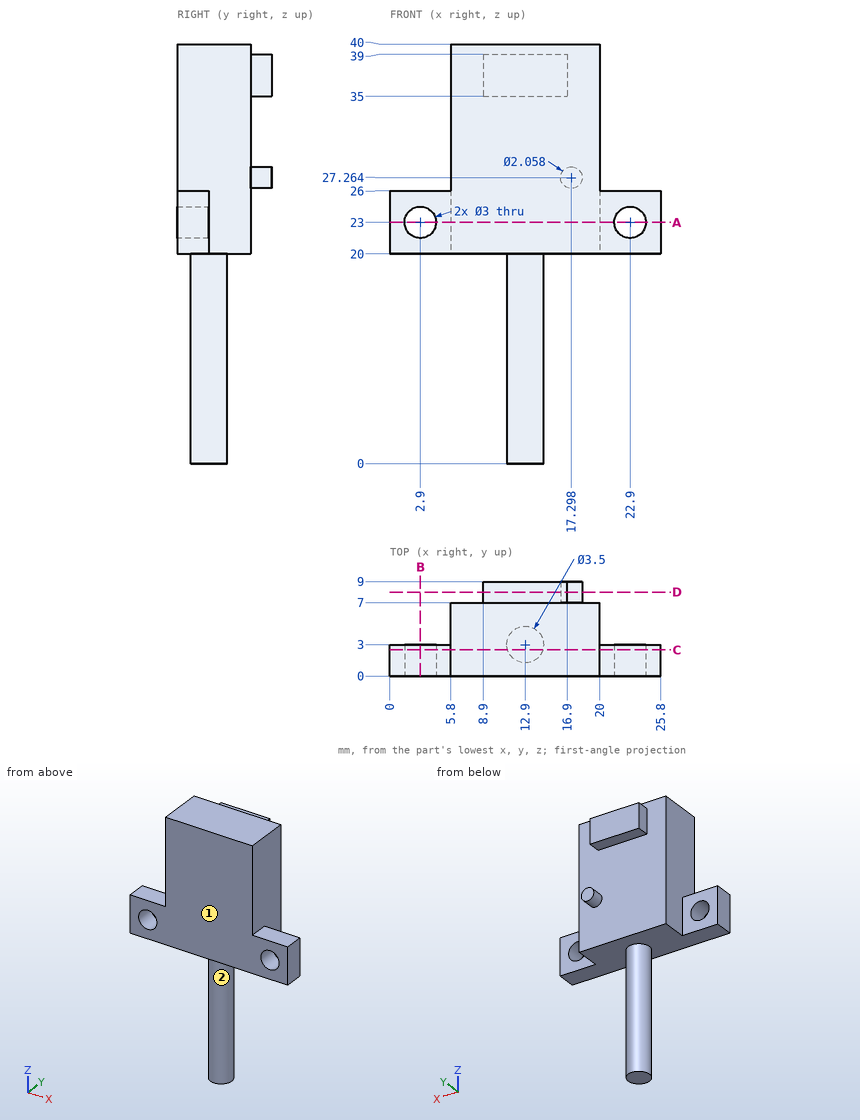
Check sheet for the drawn part. Datum: minimum x, y, z corner. Units: mm. A direction names the side the tool comes from. Coordinates: 2 decimals unless noted, no trailing zeros. Order: outer loops, then holes, each group sorted by start corner. A loop starts at its lowest first (then second) coordinate and runs counter-clockwise, first axis right, second up. Notation, with made-up numbers: M 60.25,22.5 L 72.25,22.5 A23 cw 72.25,35.5 Z; hole C 32,54 d6. An arc over 180 degrees is marked long. One line per question, with ' | ' between items. Start each with the question number.
Item 1: Sectioned sample at B-B on x = 2.9. Record the cut outline in (y, z).
Item 2: Gauge pin test, flat ends, axial feed: P1, Ø4.5, axis at x = 24.5, z = 23.5, coming from the +Y side; P2, Ø0.6, axis at x = 13, y = 7.5, coming from the -Z side; P3, Ø2.5, axis at x = 23.5, y = 1, coming from the +Z side. Record the tip position at first contact, or that the pin passes through.
Item 3: Material ranges on line 1 (X direction, y = 1.4, z = 23); line 2 (X direction, y = 0.75, z = 23.5) (1 decimal); line 3 (Z direction, x = 22.75, y = 1), recorded low to high.
Item 4: Sectioned sample at D-D on y = 8. Record the cut outline in (x, z).
Item 5: Sectioned sample at A-A on z = 23. Record the cut outline in (x, y), and give its area (3 significant figures).
Item 6: Sectioned sample at C-C on y = 2.5. Record the cut outline in (x, z).
Item 7: Access from +Z, -Z, +X, -X, +Y, -Y to the whole of each face (thin tool, end or side, straight path). Record for the marked faces 1 and 2.
Answer below:
1) outline: M 0,20 L 3,20 L 3,21.5 L 0,21.5 Z; M 0,24.5 L 3,24.5 L 3,26 L 0,26 Z
2) P1: stops at y = 3 | P2: stops at z = 35 | P3: stops at z = 26
3) line 1: x = 0 to 1.4, 4.4 to 21.4, 24.4 to 25.8 | line 2: x = 0 to 1.5, 4.3 to 21.5, 24.3 to 25.8 | line 3: z = 20 to 21.51, 24.49 to 26
4) outline: M 8.9,35 L 16.9,35 L 16.9,39 L 8.9,39 Z; C 17.3,27.26 d2.06
5) outline: M 0,0 L 1.4,0 L 1.4,3 L 0,3 Z; M 4.4,0 L 21.4,0 L 21.4,3 L 20,3 L 20,7 L 5.8,7 L 5.8,3 L 4.4,3 Z; M 24.4,0 L 25.8,0 L 25.8,3 L 24.4,3 Z | area: 116 mm^2
6) outline: M 0,20 L 11.22,20 L 11.22,0 L 14.58,0 L 14.58,20 L 25.8,20 L 25.8,26 L 20,26 L 20,40 L 5.8,40 L 5.8,26 L 0,26 Z; hole C 2.9,23 d3; hole C 22.9,23 d3
7) face 1: +Z, -Z, +X, -X, -Y | face 2: -Z
